```python
from build123d import *

# Parameters (mm, degrees)
SKETCH2_R           = 2.5
BOSS_EXTRUDE1_DEPTH = 5
SKETCH3_R           = 5
SKETCH3_R_2         = 2.5
BOSS_EXTRUDE2_DEPTH = 8
FILLET1_R           = 5


with BuildPart() as part:
    # Sketch2 → Boss-Extrude1 (new body)
    with BuildSketch(Plane(origin=(0, 0, 0), x_dir=(1, 0, 0), z_dir=(0, 1, 0))):
        with BuildLine():
            Line((-39.678172905, -46.603392635), (-19.002648889, -33))
            Line((-19.002648889, -33), (19.002648889, -33))
            Line((19.002648889, -33), (39.678172905, -46.603392635))
            ThreePointArc((39.678172905, -46.603392635), (46.603392635, -45.174640837), (45.174640837, -38.249421108))
            Line((45.174640837, -38.249421108), (21.997351111, -23))
            Line((21.997351111, -23), (-21.997351111, -23))
            Line((-21.997351111, -23), (-45.174640837, -38.249421108))
            ThreePointArc((-45.174640837, -38.249421108), (-46.603392635, -45.174640837), (-39.678172905, -46.603392635))
        make_face()
        with Locations(Location((-42.426406871, -42.426406871, 0), (0, 0, 270))):
            Circle(SKETCH2_R, mode=Mode.SUBTRACT)
        with Locations(Location((-20.5, -28, 0), (0, 0, 270))):
            Circle(SKETCH2_R, mode=Mode.SUBTRACT)
        with Locations(Location((20.5, -28, 0), (0, 0, 270))):
            Circle(SKETCH2_R, mode=Mode.SUBTRACT)
        with Locations(Location((42.426406871, -42.426406871, 0), (0, 0, 270))):
            Circle(SKETCH2_R, mode=Mode.SUBTRACT)
    extrude(amount=BOSS_EXTRUDE1_DEPTH)

    # Sketch3 → Boss-Extrude2 (add)
    # profile 1 of 2: a face of its own
    with BuildSketch(Plane(origin=(0, 5, 0), x_dir=(1, 0, 0), z_dir=(0, 1, 0))):
        with Locations(Location((-20.5, -28, 0), (0, 0, 90))):
            Circle(SKETCH3_R)
        with Locations(Location((-20.5, -28, 0), (0, 0, 270))):
            Circle(SKETCH3_R_2, mode=Mode.SUBTRACT)
    # profile 2 of 2: a face of its own
    with BuildSketch(Plane(origin=(0, 5, 0), x_dir=(1, 0, 0), z_dir=(0, 1, 0))):
        with Locations(Location((20.5, -28, 0), (0, 0, 90))):
            Circle(SKETCH3_R)
        with Locations(Location((20.5, -28, 0), (0, 0, 270))):
            Circle(SKETCH3_R_2, mode=Mode.SUBTRACT)
    extrude(amount=BOSS_EXTRUDE2_DEPTH)

    # Fillet1
    # the kernel refuses this fillet: 5 mm, written as the material it takes off along each edge
    with BuildSketch(Plane(origin=(21.997351111, -3.743377778, 23), x_dir=(0.8353971526785962, 0, 0.5496467932195132), z_dir=(0, 1, 0)), Plane(origin=(-21.997351111, -3.743377778, 23), x_dir=(1, 0, 0), z_dir=(0, 1, 0))) as fillet1_piece_1:
        with BuildLine():
            CenterArc((FILLET1_R * 0.299470222244, -FILLET1_R), FILLET1_R, 90, 33.342784883)
            Line((-FILLET1_R * 0.250176570975, -FILLET1_R * 0.164602847321), (0, 0))
            Line((0, 0), (FILLET1_R * 0.299470222244, 0))
        make_face()
    extrude(amount=12.486755556, mode=Mode.SUBTRACT)


solid = part.part
```
Can you work these out from the model? Positions are in its coordinate system, mm. A direction names the side the tool comes from. Give positions to 0.01 mm unless a question says otherwise; leave off trailing zeros. Write each loop counter-clockwise with the first axis right and the second up, starting at its lowest first coordinate (ties: lowest second). Pieces come first, ordered by that corner, then holes. Notation, with made-up numbers: (-6.5, -2.5) -> (15.5, -2.5) arc R30 ccw to (15.5, 31.5) -> close; hole circle Ø7 at (-5.75, 82). An arc over 180 degrees is marked (long way). Write item = value, one per line.
(1) I need wall thicknesses on probe 1 along X at (y, z) = (5.5, 28); probe 2 along X at (y, z) = (7, 27); probe 3 along X at (y, z) = (3.5, 29). Which ranges of each line are inside material? Lowest first, please. Write a range as from..to.
Worked out:
probe_1 = -25.5..-23, -18..-15.5, 15.5..18, 23..25.5
probe_2 = -25.4..-22.79, -18.21..-15.6, 15.6..18.21, 22.79..25.4
probe_3 = -31.12..-22.79, -18.21..18.21, 22.79..31.12
(2) Suppose I cut it at D-D on z = 42.75. Write out the boundary of the cut face in (x, y), then the cut area to 3 significant figures.
Worked out:
outline = (-47.42, 0) -> (-44.91, 0) -> (-44.91, 5) -> (-47.42, 5) -> close; (-39.95, 0) -> (-33.82, 0) -> (-33.82, 5) -> (-39.95, 5) -> close; (33.82, 0) -> (39.95, 0) -> (39.95, 5) -> (33.82, 5) -> close; (44.91, 0) -> (47.42, 0) -> (47.42, 5) -> (44.91, 5) -> close
area = 86.4 mm^2
(3) For faces 5 (the face through (29.2, 2.46, 39.71)), 6 (the face through (-22, 9.3, 23.23)), 7 (the face through (0, 2, 23)), which set-ups out of +Z, -Z, +X, -X, +Y, -Y let a thin tool reach every point of the face, with its end or its side?
Worked out:
face_5 = +Z, +Y, -Y
face_6 = +Y
face_7 = -Z, +X, -X, +Y, -Y
(4) Suppose I cut it at B-B on y = 6. Write out the boundary of the cut face in (x, z).
Worked out:
outline = circle Ø10 at (-20.5, 28); circle Ø10 at (20.5, 28); hole circle Ø5 at (-20.5, 28); hole circle Ø5 at (20.5, 28)
(5) Thinking about a two-plate mould opening in X: for faces 1 (the face through (-34.058, 2.465, 30.935)), 2 (the face through (18, 13, 27)), 3 (the face through (34.365, 2.465, 31.137)), 4 (the face through (-40.32, 2.46, 43.77)), which applies, released by +X, released by -X, zero draft, split by the parting line, or undercut?
Worked out:
face_1 = released by -X
face_2 = zero draft
face_3 = released by +X
face_4 = undercut
(6) I'm going to push flat-ended pins straight in: P1, Ø1.5, axis at x = 36.5, z = 45, coming from the +Y side; P2, Ø5.5, axis at x = 7, y = 2, coming from the +Z side; P3, Ø2, axis at y = 3, z = 30, coming from the +X side. Where does each tip first touch, or does it pass through?
Worked out:
P1 = 5
P2 = 33
P3 = 34.16
(7) Suppose I cut it at C-C on z = 35.25. Write out the boundary of the cut face in (x, y), then the cut area to 3 significant figures.
Worked out:
outline = (-40.62, 0) -> (-22.42, 0) -> (-22.42, 5) -> (-40.62, 5) -> close; (22.42, 0) -> (40.62, 0) -> (40.62, 5) -> (22.42, 5) -> close
area = 182 mm^2
(8) Suppose I cut it at A-A on z = 28. Write out the boundary of the cut face in (x, y).
Worked out:
outline = (-29.6, 0) -> (-23, 0) -> (-23, 13) -> (-25.5, 13) -> (-25.5, 5) -> (-29.6, 5) -> close; (-18, 0) -> (18, 0) -> (18, 13) -> (15.5, 13) -> (15.5, 5) -> (-15.5, 5) -> (-15.5, 13) -> (-18, 13) -> close; (23, 0) -> (29.6, 0) -> (29.6, 5) -> (25.5, 5) -> (25.5, 13) -> (23, 13) -> close
